Geometry check sheet. Reference: the model listing, model coordinates, mm. Give positions to 0.01 mm unless a question says otherwise; leave off trailing zeros.
from build123d import *

# Parameters (mm, degrees)
SKETCH_1_W          = 320
SKETCH_1_H          = 290
SKETCH_1_R          = 2.65
SKETCH_1_R_2        = 3.2
EXTRUDE_3_DEPTH     = 10
SKETCH_5_R          = 5.25
CUT_EXTRUDE_1_DEPTH = 6


with BuildPart() as part:
    # Эскиз1 → Бобышка-Вытянуть3 (new body)
    with BuildSketch(Plane(origin=(0, 0, 0), x_dir=(1, 0, 0), z_dir=(0, 1, 0))):
        Rectangle(SKETCH_1_W, SKETCH_1_H)
        with Locations((-85, 65)):
            Circle(SKETCH_1_R, mode=Mode.SUBTRACT)
        with Locations((85, 65)):
            Circle(SKETCH_1_R, mode=Mode.SUBTRACT)
        with Locations((85, -65)):
            Circle(SKETCH_1_R, mode=Mode.SUBTRACT)
        with Locations((-85, -65)):
            Circle(SKETCH_1_R, mode=Mode.SUBTRACT)
        with Locations((-147.5, 130)):
            Circle(SKETCH_1_R_2, mode=Mode.SUBTRACT)
        with Locations((-107.5, 130)):
            Circle(SKETCH_1_R_2, mode=Mode.SUBTRACT)
        with Locations((-107.5, 90)):
            Circle(SKETCH_1_R_2, mode=Mode.SUBTRACT)
        with Locations((-147.5, 90)):
            Circle(SKETCH_1_R_2, mode=Mode.SUBTRACT)
        with Locations((-147.5, -90)):
            Circle(SKETCH_1_R_2, mode=Mode.SUBTRACT)
        with Locations((-107.5, -90)):
            Circle(SKETCH_1_R_2, mode=Mode.SUBTRACT)
        with Locations((-107.5, -130)):
            Circle(SKETCH_1_R_2, mode=Mode.SUBTRACT)
        with Locations((-147.5, -130)):
            Circle(SKETCH_1_R_2, mode=Mode.SUBTRACT)
        with Locations((147.5, -130)):
            Circle(SKETCH_1_R_2, mode=Mode.SUBTRACT)
        with Locations((107.5, -130)):
            Circle(SKETCH_1_R_2, mode=Mode.SUBTRACT)
        with Locations((107.5, -90)):
            Circle(SKETCH_1_R_2, mode=Mode.SUBTRACT)
        with Locations((147.5, -90)):
            Circle(SKETCH_1_R_2, mode=Mode.SUBTRACT)
        with Locations((147.5, 90)):
            Circle(SKETCH_1_R_2, mode=Mode.SUBTRACT)
        with Locations((107.5, 90)):
            Circle(SKETCH_1_R_2, mode=Mode.SUBTRACT)
        with Locations((107.5, 130)):
            Circle(SKETCH_1_R_2, mode=Mode.SUBTRACT)
        with Locations((147.5, 130)):
            Circle(SKETCH_1_R_2, mode=Mode.SUBTRACT)
        with Locations((142, 25)):
            Circle(SKETCH_1_R_2, mode=Mode.SUBTRACT)
        with Locations((118, 25)):
            Circle(SKETCH_1_R_2, mode=Mode.SUBTRACT)
        with Locations((118, -25)):
            Circle(SKETCH_1_R_2, mode=Mode.SUBTRACT)
        with Locations((142, -25)):
            Circle(SKETCH_1_R_2, mode=Mode.SUBTRACT)
    extrude(amount=EXTRUDE_3_DEPTH)

    # Эскиз5 → Вырез-Вытянуть1 (cut)
    with BuildSketch(Plane.XZ):
        with Locations((-147.5, 130)):
            Circle(SKETCH_5_R)
        with Locations((-107.5, 130)):
            Circle(SKETCH_5_R)
        with Locations((-107.5, 90)):
            Circle(SKETCH_5_R)
        with Locations((-147.5, 90)):
            Circle(SKETCH_5_R)
        with Locations((-147.5, -90)):
            Circle(SKETCH_5_R)
        with Locations((-107.5, -90)):
            Circle(SKETCH_5_R)
        with Locations((-107.5, -130)):
            Circle(SKETCH_5_R)
        with Locations((-147.5, -130)):
            Circle(SKETCH_5_R)
        with Locations((147.5, -130)):
            Circle(SKETCH_5_R)
        with Locations((107.5, -130)):
            Circle(SKETCH_5_R)
        with Locations((107.5, -90)):
            Circle(SKETCH_5_R)
        with Locations((147.5, -90)):
            Circle(SKETCH_5_R)
        with Locations((147.5, 90)):
            Circle(SKETCH_5_R)
        with Locations((107.5, 90)):
            Circle(SKETCH_5_R)
        with Locations((107.5, 130)):
            Circle(SKETCH_5_R)
        with Locations((147.5, 130)):
            Circle(SKETCH_5_R)
        with Locations((142, 25)):
            Circle(SKETCH_5_R)
        with Locations((118, 25)):
            Circle(SKETCH_5_R)
        with Locations((118, -25)):
            Circle(SKETCH_5_R)
        with Locations((142, -25)):
            Circle(SKETCH_5_R)
    extrude(amount=-CUT_EXTRUDE_1_DEPTH, mode=Mode.SUBTRACT)


solid = part.part
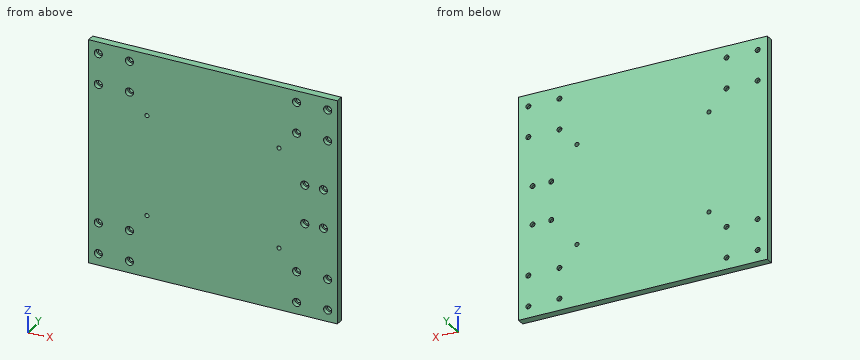
Item 1: Gauge pin test, flat ends, axial feed: pin 1 (7.5 mm diameter, centred on x = -147.5, z = 130, fed in from -Y); pin 2 (5 mm diameter, centred on x = -107.5, z = -130, fed in from +Y). Record the tip position at first contact, or that the pin passes through.
Reported:
pin 1: stops at y = 6
pin 2: passes through
Item 2: Sectioned sample at A-A (y = 4.25). Give the number of separate pieces and of enclosed holes in the cut face, and give its area (3 significant figures).
Reported:
separate pieces: 1
enclosed holes: 24
area: 91,000 mm2
Item 3: Scan lines: L1, parallel to Z at x = 107.5, y = 8.15; L2, parallel to Z at x = -147.5, y = 4.15; L3, parallel to X at y = 4.25, z = -65. Record each from-to range of solid material in increasing order.
Reported:
L1: z = -145 to -133.2, -126.8 to -93.2, -86.8 to 86.8, 93.2 to 126.8, 133.2 to 145
L2: z = -145 to -135.25, -124.75 to -95.25, -84.75 to 84.75, 95.25 to 124.75, 135.25 to 145
L3: x = -160 to -87.65, -82.35 to 82.35, 87.65 to 160
